The model under review builds one solid part; all positions refer to its coordinate system, in mm. Give positions to 0.01 mm unless a question says otherwise; leave off trailing zeros. Write item = value, one per line. Start each with the question number.
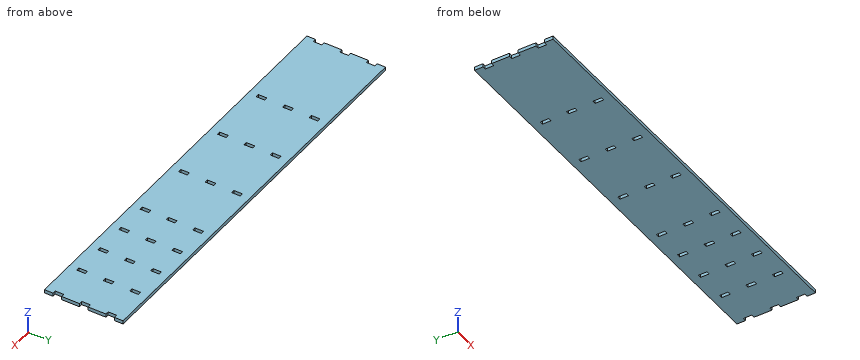
```python
from build123d import *

# Parameters (mm, degrees)
F0_W     = 287
F0_H     = 55
F1_DEPTH = 2.4
F2_W     = 2.4
F2_H     = 6
F3_DEPTH = 2.401


with BuildPart() as f1:
    # F0 (on Top) → F1 (new body)
    with BuildSketch(Plane.XY):
        Rectangle(F0_W, F0_H)
    extrude(amount=F1_DEPTH)

    # F2 (on face) → F3 (cut, through all)
    with BuildSketch(Plane.XY.offset(2.4)):
        with Locations((-142.3, 0)):
            Rectangle(F2_W, F2_H)
        with Locations((-142.3, -18.5)):
            Rectangle(F2_W, F2_H)
        with Locations((-142.3, 18.5)):
            Rectangle(F2_W, F2_H)
        with Locations((-79.9, 18.5)):
            Rectangle(F2_W, F2_H)
        with Locations((-79.9, 0)):
            Rectangle(F2_W, F2_H)
        with Locations((-79.9, -18.5)):
            Rectangle(F2_W, F2_H)
        with Locations((-37.5, -18.5)):
            Rectangle(F2_W, F2_H)
        with Locations((-37.5, 0)):
            Rectangle(F2_W, F2_H)
        with Locations((-37.5, 18.5)):
            Rectangle(F2_W, F2_H)
        with Locations((4.9, 18.5)):
            Rectangle(F2_W, F2_H)
        with Locations((4.9, 0)):
            Rectangle(F2_W, F2_H)
        with Locations((4.9, -18.5)):
            Rectangle(F2_W, F2_H)
        with Locations((47.3, -18.5)):
            Rectangle(F2_W, F2_H)
        with Locations((47.3, 0)):
            Rectangle(F2_W, F2_H)
        with Locations((47.3, 18.5)):
            Rectangle(F2_W, F2_H)
        with Locations((70.3, 18.5)):
            Rectangle(F2_W, F2_H)
        with Locations((70.3, 0)):
            Rectangle(F2_W, F2_H)
        with Locations((70.3, -18.5)):
            Rectangle(F2_W, F2_H)
        with Locations((93.3, -18.5)):
            Rectangle(F2_W, F2_H)
        with Locations((93.3, 0)):
            Rectangle(F2_W, F2_H)
        with Locations((93.3, 18.5)):
            Rectangle(F2_W, F2_H)
        with Locations((116.3, 18.5)):
            Rectangle(F2_W, F2_H)
        with Locations((116.3, 0)):
            Rectangle(F2_W, F2_H)
        with Locations((116.3, -18.5)):
            Rectangle(F2_W, F2_H)
        with Locations((142.3, 18.5)):
            Rectangle(F2_W, F2_H)
        with Locations((142.3, 0)):
            Rectangle(F2_W, F2_H)
        with Locations((142.3, -18.5)):
            Rectangle(F2_W, F2_H)
    extrude(amount=-F3_DEPTH, mode=Mode.SUBTRACT)


solid = f1.part
```
Item 1: Clearance check with flat-ended pins moving along their axes: P1, Ø1.2, axis at y = 0.5, z = 1.5, coming from the +X side; P2, Ø1.2, axis at y = 0, z = 1.5, coming from the -X side. State where each tip first meets the part, or that it passes through.
Item 2: We need section A-A, the plane y = -19. Give the number of separate pieces and of enclosed holes in the cut face, and give its area (3 significant figures).
Item 3: To check wall thickness, follow probe 1 along Y at (x, z) = (-79, 0.45). State the ranges of the line that lie inside material, in increasing order. Write a range as [from, to].
Worked out:
q1.P1 = 141.1
q1.P2 = -141.1
q2.separate_pieces = 8
q2.enclosed_holes = 0
q2.area = 637 mm²
q3.probe_1 = [-27.5, -21.5], [-15.5, -3], [3, 15.5], [21.5, 27.5]
